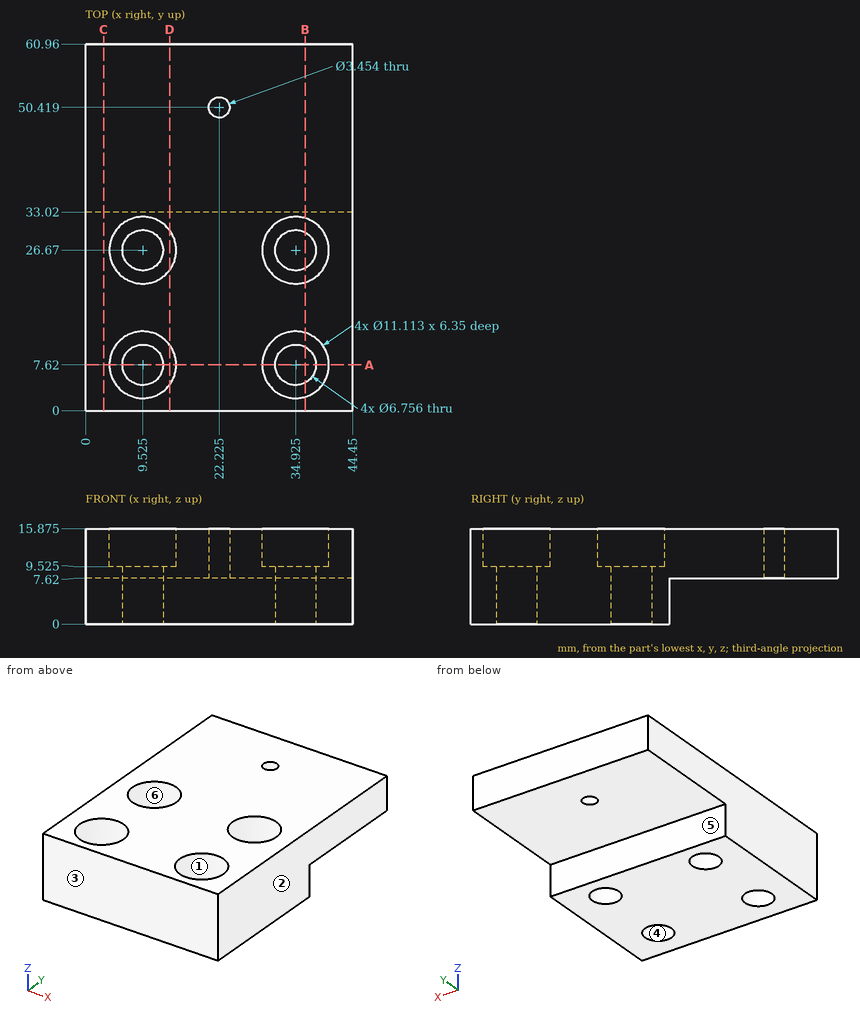
Verification items for this drawing (mm, ordinates from the low corner). A direction names the side the tool comes from. Coordinates: 2 decimals unless noted, no trailing zeros. Write each loop counter-clockwise with the first axis right and the second up, starting at its lowest first coordinate (ties: lowest second). Pieces come first, ordered by that corner, then holes. Notation, with made-up numbers: (44.25, 34.5) -> (100.25, 34.5) arc R27 cw to (100.25, 69.5) -> close; hole circle Ø2 at (44.5, 83). An arc over 180 degrees is marked (long way). One line per item, written item: value. Start each with the question number.
Q1. Cross-section at A-A on y = 7.62. State how many separate pieces and enclosed holes the cut face has, and give its area (3 significant figures).
Q2. Access from +Z, -Z, +X, -X, +Y, -Y to the whole of each face (thin tool, end or side, straight path). Record for the marked faces 4, 5 and 6.
Q3. Cross-section at C-C on x = 3. Enter the section's corners in (y, z) (1 decimal).
Q4. Cross-section at B-B on x = 36.5. Enter the section's corners in (y, z) (1 decimal).
Q5. Thickness scan on L1, parallel to X at y = 6, z = 14; L2, parallel to X at y = 29, z = 11; L3, parallel to Y at x = 32, z = 11.75 (1 decimal). Record the ranges inside material, lowest first. Write a range as from..to.
Q6. Go/stop test with flat-tipped pins: P1, Ø5.5, axis at x = 32.5, y = 7, coming from the +Z side (1 decimal); P2, Ø12, axis at x = 6.5, y = 51.5, coming from the -Z side; P3, Ø6, axis at x = 28, z = 4, coming from the +Y side. Record where each tip stops, or that it passes through.
Q7. Mould release check, pull along Y, two halves, no side actions. Record for the marked faces 1, 2 and 3: pulls with the +Y half, pulls with the -Y half, needs draft (parallel to the pull), parting line crosses it, or undercut.
Q8. Cross-section at D-D on x = 14. Enter the section's corners in (y, z) (1 decimal).
Checked values:
1. separate pieces: 3
1. enclosed holes: 0
1. area: 436 mm²
2. face 4: +Z, -Z
2. face 5: -Z, +X, -X, +Y
2. face 6: +Z
3. outline: (0, 0) -> (33, 0) -> (33, 7.6) -> (61, 7.6) -> (61, 15.9) -> (0, 15.9) -> close
4. outline: (0, 0) -> (4.6, 0) -> (4.6, 9.5) -> (2.3, 9.5) -> (2.3, 15.9) -> (0, 15.9) -> close; (10.6, 0) -> (23.7, 0) -> (23.7, 9.5) -> (21.3, 9.5) -> (21.3, 15.9) -> (12.9, 15.9) -> (12.9, 9.5) -> (10.6, 9.5) -> close; (29.7, 0) -> (33, 0) -> (33, 7.6) -> (61, 7.6) -> (61, 15.9) -> (32, 15.9) -> (32, 9.5) -> (29.7, 9.5) -> close
5. L1: x = 0..4.21, 14.84..29.61, 40.24..44.45
5. L2: x = 0..4.48, 14.57..29.88, 39.97..44.45
5. L3: y = 0..2.9, 12.3..21.9, 31.4..61
6. P1: stops at z = 9.5
6. P2: stops at z = 7.62
6. P3: stops at y = 33.02
7. face 1: undercut
7. face 2: needs draft
7. face 3: pulls with the -Y half
8. outline: (0, 0) -> (33, 0) -> (33, 7.6) -> (61, 7.6) -> (61, 15.9) -> (30, 15.9) -> (30, 9.5) -> (23.4, 9.5) -> (23.4, 15.9) -> (10.9, 15.9) -> (10.9, 9.5) -> (4.3, 9.5) -> (4.3, 15.9) -> (0, 15.9) -> close
